Verification items for the finished model (mm, model axes). A direction names the side the tool comes from. Coordinates: 2 decimals unless noted, no trailing zeros. Order: outer loops, then holes, each group sorted by start corner. A loop starts at its lowest first (then second) coordinate and runs counter-clockwise, first axis right, second up. Notation, with made-up numbers: M 9.5,10 L 68.5,10 A28 cw 68.5,34 Z; hole C -2,51.25 d2. An arc over 180 degrees is marked long. Use one line per item in the form item = value. Start each with the question number.
```python
from build123d import *

# Parameters (mm, degrees)
BOSS_EXTRUDE1_DEPTH = 76.2
SKETCH3_R           = 6.35
BOSS_EXTRUDE2_DEPTH = 7.9375
SKETCH4_R           = 6.35
BOSS_EXTRUDE3_DEPTH = 7.9375


with BuildPart() as part:
    # Sketch1 → Boss-Extrude1 (new body)
    with BuildSketch(Plane(origin=(0, 0, 0), x_dir=(1, 0, 0), z_dir=(0, 1, 0))):
        Polygon((5.948792794, 4.286630102), (-0.737934168, 7.295120732), (-6.686726962, 3.008490631), (-5.948792794, -4.286630102), (0.737934168, -7.295120732), (6.686726962, -3.008490631), align=None)
    extrude(amount=BOSS_EXTRUDE1_DEPTH)

    # Sketch3 → Boss-Extrude2 (add)
    with BuildSketch(Plane(origin=(0, 0, 0), x_dir=(-1, 0, 0), z_dir=(0, -1, 0))):
        Circle(SKETCH3_R)
    extrude(amount=BOSS_EXTRUDE2_DEPTH)

    # Sketch4 → Boss-Extrude3 (add)
    with BuildSketch(Plane(origin=(0, 76.2, 0), x_dir=(1, 0, 0), z_dir=(0, 1, 0))):
        Circle(SKETCH4_R)
    extrude(amount=BOSS_EXTRUDE3_DEPTH)


solid = part.part
```
1. Cross-section at A-A on y = 45. Enter the section's corners in (x, z).
2. Release check for a two-part mould opening along X. For faces 5 (the flat face through (-3.67, 37.57, -5.18)), 6 (the cylindrical face through (-1.38, 80.11, 6.2)), 7 (the flat face through (-5.3, 76.2, 3.8)), 8 (the flat face through (2.65, 37.57, -5.77)) record: pulls with the +X half, pulls with the -X half, needs draft (parallel to the pull), parting line crosses it, or undercut.
3. Material ranges on line 1 along X through (y, z) = (62, 3); line 2 along Z through (x, y) = (1.75, 47); line 3 along X through (y, z) = (65.5, 5.75), recorded low to high.
4. Tool access check on faces 1 (the flat face through (-5.3, 0, 3.8)), 2 (the flat face through (-2.65, 37.57, 5.77)), 3 (the cylindrical face through (1.38, -3.91, 6.2)), 4 (the flat face through (5.3, 0, -3.8)). Record the directions out of +Z, -Z, +X, -X, +Y, -Y that give a thin tool (end or side, any length) a straight path to the whole face; none if there is none.
5. Depth check by flat-ended pin: P1, Ø5, axis at x = 4, y = 28, coming from the -Z side; P2, Ø1.5, axis at x = -3, y = 22, coming from the +Z side; P3, Ø1.1, axis at x = 2, z = 6.5, coming from the -Y side; P4, Ø2, axis at y = 39, z = 0, coming from the -X side. Enter the tip coordinate at first touch or a pass-through.
Final values:
q1.outline = M -6.69,-3.01 L -0.74,-7.3 L 5.95,-4.29 L 6.69,3.01 L 0.74,7.3 L -5.95,4.29 Z
q2.face_5 = pulls with the -X half
q2.face_6 = parting line crosses it
q2.face_7 = needs draft
q2.face_8 = pulls with the +X half
q3.line_1 = -6.08 to 6.69
q3.line_2 = -6.18 to 6.57
q3.line_3 = -2.7 to 2.88
q4.face_1 = +Z, -X, -Y
q4.face_2 = +Z, -X, +Y, -Y
q4.face_3 = -Y
q4.face_4 = -Z, +X, -Y
q5.P1 = -6.29
q5.P2 = 5.95
q5.P3 = -7.94
q5.P4 = -6.48
